For this review, take the finished solid that the model builds, in its own axes (mm). A direction names the side the tool comes from. Round coordinates to 2 decimals unless told otherwise and drop trailing zeros. Write each loop counter-clockwise with the first axis right and the second up, starting at its lowest first coordinate (ties: lowest second). Pieces come first, ordered by that corner, then holes. Notation, with made-up numbers: (76, 87) -> (103, 87) arc R7 cw to (103, 98) -> close; hole circle Ø5 at (30.25, -16.5). An arc over 180 degrees is marked (long way). Answer in a Markdown table with one row per item.
from build123d import *

# Parameters (mm, degrees)
F2_SIZE2 = 2
F2_SIZE  = 3.4641016151


with BuildPart() as f1:
    # F0 (on Front) → F1 (revolve)
    with BuildSketch(Plane.XZ):
        with BuildLine():
            Line((-47.1474705863, -2.0639507875), (-45.5, -2.0639507875))
            Line((-45.5, -2.0639507875), (-41.5, -2.0639507875))
            Line((-41.5, -2.0639507875), (-41.5, 80.4360492125))
            Line((-41.5, 80.4360492125), (-45.5, 80.4360492125))
            Line((-45.5, 80.4360492125), (-45.5, 18.9360492125))
            Line((-45.5, 18.9360492125), (-45.5, 7.5360492125))
            Line((-45.5, 7.5360492125), (-53.0143515468, 2.7360492125))
            Line((-53.0143515468, 2.7360492125), (-53.0143515468, -2.0639507875))
            Line((-53.0143515468, -2.0639507875), (-49.8812325073, -2.0639507875))
            ThreePointArc((-49.8812325073, -2.0639507875), (-48.5143515468, -0.697069827), (-47.1474705863, -2.0639507875))
        make_face()
        with BuildLine():
            Line((-45.5, 80.4360492125), (-41.5, 80.4360492125))
            Line((-41.5, 80.4360492125), (-41.5, 162.9360492125))
            Line((-41.5, 162.9360492125), (-45.5, 162.9360492125))
            Line((-45.5, 162.9360492125), (-47.1474705863, 162.9360492125))
            ThreePointArc((-47.1474705863, 162.9360492125), (-48.5143515468, 161.569168252), (-49.8812325073, 162.9360492125))
            Line((-49.8812325073, 162.9360492125), (-53.0143515468, 162.9360492125))
            Line((-53.0143515468, 162.9360492125), (-53.0143515468, 158.1360492125))
            Line((-53.0143515468, 158.1360492125), (-45.5, 153.3360492125))
            Line((-45.5, 153.3360492125), (-45.5, 141.9360492125))
            Line((-45.5, 141.9360492125), (-45.5, 80.4360492125))
        make_face()
    revolve(axis=Axis((0, 0, 19.3934533745), (0, 0, 1)))

    # F2
    f2_edges = [f1.edges().sort_by_distance(p)[0] for p in [
        (41.5, 0, 162.936049),
        (41.5, 0, -2.063951),
    ]]
    f2_side = f1.faces().sort_by_distance((41.5, 0, 80.436049))[0]
    chamfer(f2_edges, length=F2_SIZE, length2=F2_SIZE2, reference=f2_side)


solid = f1.part
1) For faces 4 (the cylindrical face through (-28.5, -44.7, 0.3)), 5 (the cylindrical face through (36.107, 27.686, 79.415)), list the 3-axis set-ups (+Z, -Z, +X, -X, +Y, -Y) from which the entire face can be reached by the end or side of a thin tool; tool diameter is ignored.
Solved:
| item | result |
|---|---|
| face 4 | +Z, -Z |
| face 5 | none |
2) Consider section C-C on z = 11. State the section outline as (x, y) points, then the cut area to 3 significant figures.
Solved:
| item | result |
|---|---|
| outline | circle Ø91 at (0, 0); hole circle Ø83 at (0, 0) |
| area | 1,090 mm² |
3) Mouldability with a two-part tool opening along Z and no side actions: class faces 1 (the cylindrical face through (-28.5, -44.7, 160.5)), 2 (the conical face through (-24.71, -38.76, 7.24)), 3 (the flat face through (-36, 35, 162.936)) as pulls with the +Z half, pulls with the -Z half, needs draft (parallel to the pull), parting line crosses it, or undercut.
Solved:
| item | result |
|---|---|
| face 1 | needs draft |
| face 2 | undercut |
| face 3 | pulls with the +Z half |
4) Clearance check with flat-ended pins moving along their axes: pin 1 Ø6 at (x, y) = (-18, 32) entering from +Z; pin 2 Ø6 at (y, z) = (10.5, 130.5) entering from +X; pin 3 Ø8 at (y, z) = (-12.5, 137.5) entering from -X; pin 4 Ø2 at (y, z) = (-19, 145.5) entering from +X. State where each tip first meets the part, or that it passes through.
Solved:
| item | result |
|---|---|
| pin 1 | through |
| pin 2 | x = 44.88 |
| pin 3 | x = -44.7 |
| pin 4 | x = 41.79 |
5) For line 1 (Y direction, x = 0, z = 98); line 2 (X direction, y = 29.5, z = 126), list the stretches that pass through material, from the lowest coordinate up. Write a range as [from, to].
Solved:
| item | result |
|---|---|
| line 1 | [-45.5, -41.5], [41.5, 45.5] |
| line 2 | [-34.64, -29.19], [29.19, 34.64] |
6) Consider section A-A on x = 0. State the section outline as (y, z) points, then the cut area to 3 significant figures.
Solved:
| item | result |
|---|---|
| outline | (-53.01, -2.06) -> (-49.88, -2.06) arc R1.37 cw to (-47.15, -2.06) -> (-43.5, -2.06) -> (-41.5, 1.4) -> (-41.5, 159.47) -> (-43.5, 162.94) -> (-47.15, 162.94) arc R1.37 cw to (-49.88, 162.94) -> (-53.01, 162.94) -> (-53.01, 158.14) -> (-45.5, 153.34) -> (-45.5, 7.54) -> (-53.01, 2.74) -> close; (41.5, 1.4) -> (43.5, -2.06) -> (47.15, -2.06) arc R1.37 cw to (49.88, -2.06) -> (53.01, -2.06) -> (53.01, 2.74) -> (45.5, 7.54) -> (45.5, 153.34) -> (53.01, 158.14) -> (53.01, 162.94) -> (49.88, 162.94) arc R1.37 cw to (47.15, 162.94) -> (43.5, 162.94) -> (41.5, 159.47) -> close |
| area | 1,510 mm² |
